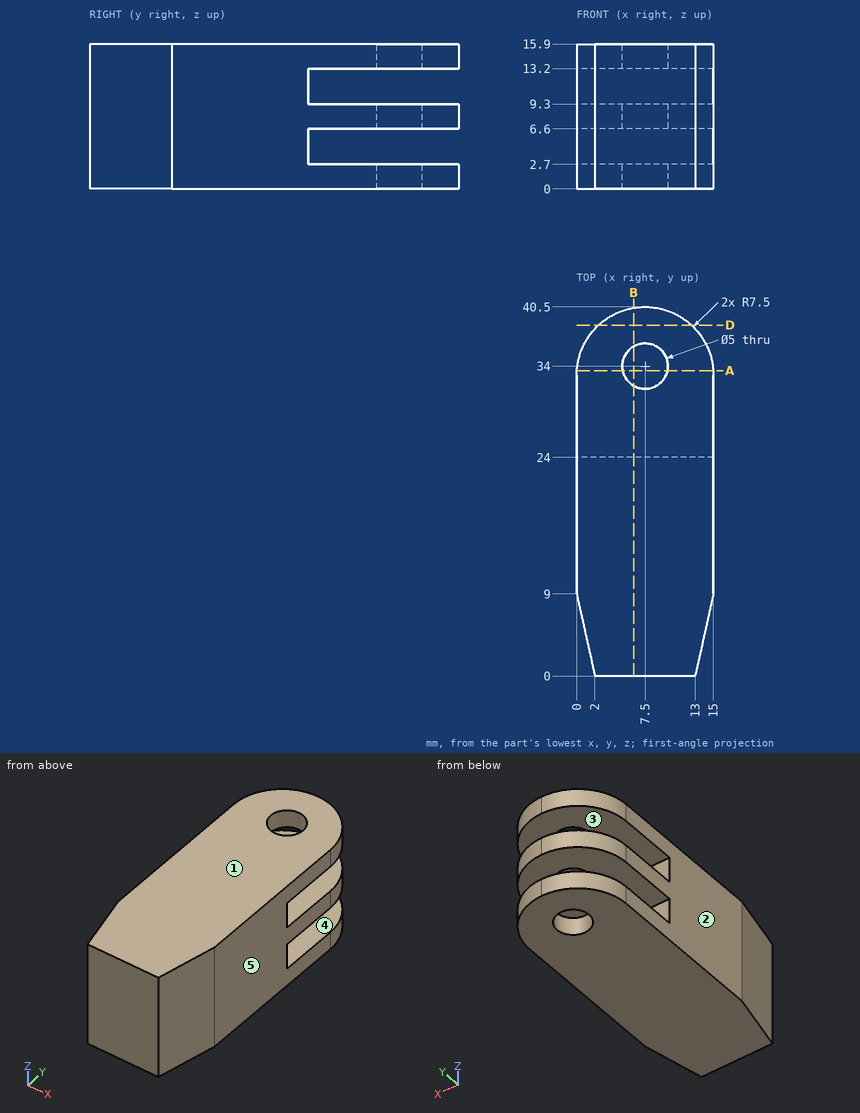
Geometry check sheet. Reference: drawing and pictorial views, mm from the part's lowest x, y, z. A direction names the side the tool comes from. Give positions to 0.01 mm unless a question says otherwise; leave off trailing zeros. Order: outer loops, then holes, each group sorted by start corner. A loop starts at its lowest first (then second) coordinate and runs counter-clockwise, first axis right, second up. Notation, with made-up numbers: (89, 59.25) -> (148, 59.25) arc R17 cw to (148, 67.25) -> close; hole circle Ø3 at (73.5, 10.5). An arc over 180 degrees is marked (long way). Write each question's results on one line, items separated by ' | '. Start each with the question number.
(1) Sectioned sample at A-A (y = 33.5). Enter the section's corners in (x, z).
(2) Scan lines: line 1 (Z direction, x = 11.5, y = 31); line 2 (Y direction, x = 7.5, z = 1.5); line 3 (Y direction, x = 2.75, z = 5). Record each from-to range of solid material in increasing order.
(3) Access from +Z, -Z, +X, -X, +Y, -Y to the whole of each face (thin tool, end or side, straight path). Record for the marked faces 4 and 5.
(4) Mould release check, pull along Z, two halves, no side actions. Record for the marked faces 1, 2 and 3: pulls with the +Z half, pulls with the -Z half, needs draft (parallel to the pull), parting line crosses it, or undercut.
(5) Gauge pin test, flat ends, axial feed: P1, Ø6, axis at x = 8.5, z = 13.5, coming from the -Y side; P2, Ø5, axis at x = 12.5, z = 10.5, coming from the +Y side (1 decimal); P3, Ø1.9, axis at x = 11, z = 12, coming from the +Y side. Record the tip position at first contact, or that the pin passes through.
(6) Sectioned sample at B-B (x = 6.25). Enter the section's corners in (y, z) (1 decimal).
(7) Sectioned sample at D-D (y = 38.5). Enter the section's corners in (x, z).
Answer below:
1) outline: (0.02, 0) -> (5.05, 0) -> (5.05, 2.7) -> (0.02, 2.7) -> close; (0.02, 6.6) -> (5.05, 6.6) -> (5.05, 9.3) -> (0.02, 9.3) -> close; (0.02, 13.2) -> (5.05, 13.2) -> (5.05, 15.9) -> (0.02, 15.9) -> close; (9.95, 0) -> (14.98, 0) -> (14.98, 2.7) -> (9.95, 2.7) -> close; (9.95, 6.6) -> (14.98, 6.6) -> (14.98, 9.3) -> (9.95, 9.3) -> close; (9.95, 13.2) -> (14.98, 13.2) -> (14.98, 15.9) -> (9.95, 15.9) -> close
2) line 1: 0 to 2.7, 6.6 to 9.3, 13.2 to 15.9 | line 2: 0 to 31.5, 36.5 to 40.5 | line 3: 0 to 24
3) face 4: +X, -X, +Y | face 5: +Z, -Z, +X, +Y, -Y
4) face 1: pulls with the +Z half | face 2: needs draft | face 3: undercut
5) P1: y = 0 | P2: y = 40 | P3: y = 24
6) outline: (0, 0) -> (31.8, 0) -> (31.8, 2.7) -> (24, 2.7) -> (24, 6.6) -> (31.8, 6.6) -> (31.8, 9.3) -> (24, 9.3) -> (24, 13.2) -> (31.8, 13.2) -> (31.8, 15.9) -> (0, 15.9) -> close; (36.2, 0) -> (40.4, 0) -> (40.4, 2.7) -> (36.2, 2.7) -> close; (36.2, 6.6) -> (40.4, 6.6) -> (40.4, 9.3) -> (36.2, 9.3) -> close; (36.2, 13.2) -> (40.4, 13.2) -> (40.4, 15.9) -> (36.2, 15.9) -> close
7) outline: (2.4, 0) -> (12.6, 0) -> (12.6, 2.7) -> (2.4, 2.7) -> close; (2.4, 6.6) -> (12.6, 6.6) -> (12.6, 9.3) -> (2.4, 9.3) -> close; (2.4, 13.2) -> (12.6, 13.2) -> (12.6, 15.9) -> (2.4, 15.9) -> close
